For this review, take the finished solid that the model builds, in its own axes (mm). A direction names the side the tool comes from. Round coordinates to 2 decimals unless told otherwise and drop trailing zeros. Write each loop counter-clockwise with the first axis right and the second up, starting at its lowest first coordinate (ties: lowest second). Pieces come first, ordered by that corner, then holes. Notation, with made-up numbers: (-11.75, 48) -> (-1.75, 48) arc R29 ccw to (-1.75, 80) -> close; hole circle Ø5 at (64, 63.25). An arc over 180 degrees is marked (long way). Answer as CSV lines item,"result". Start each with the question number.
Item 1: Machinability: for faces 1 (the flat face through (-12, -1, 4.5)), 2 (the conical face through (-38.13, -18.06, 7.87)), 3 (the cylindrical face through (-28.784, 16.818, 2.885)), which of the approach directions +Z, -Z, +X, -X, +Y, -Y give a long, thin tool a straight path to every point of the face, cutting with its end or side? Answer none if there is none.
Item 2: For pin 1 Ø3 at (y, z) = (12, 4) entering from -X; pin 2 Ø2.5 at (x, z) = (30, 4) entering from +Y; pin 3 Ø4 at (x, y) = (-15, -2) entering from -Z, all flat-tipped, find the tip position at first contact; note any pin that passes through.
Item 3: Mouldability with a two-part tool opening along X and no side actions: class faces 4 (the cylindrical face through (0.4, 13.9, 5.6)), 5 (the conical face through (38.06, -18.13, 7.87)), 6 (the conical face through (-38.12, -18.06, 0.12)), 7 (the cylindrical face through (-18, 0, 6)) as +X half, -X half, draft (parallel to the pull), parting line (faces both ways), or undercut.
Item 4: Take a section at B-B on x = 15. Give the boundary of the cut face in (y, z), then the cut area to 3 significant figures.
Item 5: Wall thickness on probe 1 along X at (y, z) = (13.75, 4); probe 2 along Y at (x, z) = (-15, 1.8); probe 3 along X at (y, z) = (-0.5, 6.25): over which ranges is each line inside the solid? List them lowest first. Write a range as from..to.
Item 6: Take a section at A-A on y = 0. Count the separate pieces of the cut face and the enclosed holes in it, then the cut area to 3 significant figures.
```python
from build123d import *

# Parameters (mm, degrees)
SKETCH1_W                             = 80
SKETCH1_H                             = 40
SKETCH1_R                             = 7
SKETCH1_R_2                           = 3
BOSS_EXTRUDE1_DEPTH                   = 8
CUT_EXTRUDE1_OUTLINE_R                = 7
CUT_EXTRUDE1_OUTLINE_R_2              = 3
CUT_EXTRUDE1_DEPTH                    = 4.5
FILLET1_R                             = 5
TAP_DRILL_FOR_M4X0_7_TAP1_D           = 3.3
TAP_DRILL_FOR_M4X0_7_TAP1_DEPTH       = 12
TAP_DRILL_FOR_M4X0_7_TAP1_CSINK_D     = 3.35
TAP_DRILL_FOR_M4X0_7_TAP1_CSINK_ANGLE = 90
TAP_DRILL_FOR_M4X0_7_TAP1_TIP         = 0.991420021
TAP_DRILL_FOR_M4X0_7_TAP2_D           = 3.3
TAP_DRILL_FOR_M4X0_7_TAP2_DEPTH       = 12
TAP_DRILL_FOR_M4X0_7_TAP2_CSINK_D     = 3.35
TAP_DRILL_FOR_M4X0_7_TAP2_CSINK_ANGLE = 90
TAP_DRILL_FOR_M4X0_7_TAP2_TIP         = 0.991420021
TAP_DRILL_FOR_M4X0_7_TAP3_D           = 3.3
TAP_DRILL_FOR_M4X0_7_TAP3_DEPTH       = 12
TAP_DRILL_FOR_M4X0_7_TAP3_CSINK_D     = 3.35
TAP_DRILL_FOR_M4X0_7_TAP3_CSINK_ANGLE = 90
TAP_DRILL_FOR_M4X0_7_TAP3_TIP         = 0.991420021
CHAMFER1_SIZE                         = 0.75


# Read off the part's stored shape, not the designer's step: Cut-Extrude1
with BuildPart() as part:
    # Sketch1 → Boss-Extrude1 (new body)
    # profile 1 of 3: a face of its own
    with BuildSketch(Plane.XY):
        Rectangle(SKETCH1_W, SKETCH1_H)
        with Locations((15, 0)):
            Circle(SKETCH1_R, mode=Mode.SUBTRACT)
        with Locations((-15, 0)):
            Circle(SKETCH1_R, mode=Mode.SUBTRACT)
    # profile 2 of 3: a face of its own
    with BuildSketch(Plane.XY):
        with Locations((-15, 0)):
            Circle(SKETCH1_R)
        with Locations((-15, 0)):
            Circle(SKETCH1_R_2, mode=Mode.SUBTRACT)
    # profile 3 of 3: a face of its own
    with BuildSketch(Plane.XY):
        with Locations((15, 0)):
            Circle(SKETCH1_R)
        with Locations((15, 0)):
            Circle(SKETCH1_R_2, mode=Mode.SUBTRACT)
    extrude(amount=BOSS_EXTRUDE1_DEPTH)

    # Cut-Extrude1 outline → Cut-Extrude1 (cut)
    # profile 1 of 2: a face of its own
    with BuildSketch(Plane.XY):
        with Locations((-15, 0)):
            Circle(CUT_EXTRUDE1_OUTLINE_R)
        with Locations((-15, 0)):
            Circle(CUT_EXTRUDE1_OUTLINE_R_2, mode=Mode.SUBTRACT)
    # profile 2 of 2: a face of its own
    with BuildSketch(Plane.XY):
        with Locations((15, 0)):
            Circle(CUT_EXTRUDE1_OUTLINE_R)
        with Locations((15, 0)):
            Circle(CUT_EXTRUDE1_OUTLINE_R_2, mode=Mode.SUBTRACT)
    extrude(amount=CUT_EXTRUDE1_DEPTH, mode=Mode.SUBTRACT)

    # Fillet1
    fillet1_edges = [part.edges().sort_by_distance(p)[0] for p in [
        (40, -20, 4),
        (-40, -20, 4),
        (-40, 20, 4),
        (40, 20, 4),
    ]]
    fillet(fillet1_edges, radius=FILLET1_R)

    # Tap Drill for M4x0.7 Tap1
    with Locations(Plane(origin=(0, 20, 0), x_dir=(1, 0, 0), z_dir=(0, 1, 0))):
        with Locations((30, -4), (0, -4), (-30, -4)):
            CounterSinkHole(TAP_DRILL_FOR_M4X0_7_TAP1_D / 2, TAP_DRILL_FOR_M4X0_7_TAP1_CSINK_D / 2, depth=TAP_DRILL_FOR_M4X0_7_TAP1_DEPTH, counter_sink_angle=TAP_DRILL_FOR_M4X0_7_TAP1_CSINK_ANGLE)
            with Locations((0, 0, -(TAP_DRILL_FOR_M4X0_7_TAP1_DEPTH + TAP_DRILL_FOR_M4X0_7_TAP1_TIP / 2))):  # 118° drill point
                Cone(0, TAP_DRILL_FOR_M4X0_7_TAP1_D / 2, TAP_DRILL_FOR_M4X0_7_TAP1_TIP, mode=Mode.SUBTRACT)

    # Tap Drill for M4x0.7 Tap2
    with Locations(Plane(origin=(40, 0, 0), x_dir=(0, 0, -1), z_dir=(1, 0, 0))):
        with Locations((-4, 12)):
            CounterSinkHole(TAP_DRILL_FOR_M4X0_7_TAP2_D / 2, TAP_DRILL_FOR_M4X0_7_TAP2_CSINK_D / 2, depth=TAP_DRILL_FOR_M4X0_7_TAP2_DEPTH, counter_sink_angle=TAP_DRILL_FOR_M4X0_7_TAP2_CSINK_ANGLE)
            with Locations((0, 0, -(TAP_DRILL_FOR_M4X0_7_TAP2_DEPTH + TAP_DRILL_FOR_M4X0_7_TAP2_TIP / 2))):  # 118° drill point
                Cone(0, TAP_DRILL_FOR_M4X0_7_TAP2_D / 2, TAP_DRILL_FOR_M4X0_7_TAP2_TIP, mode=Mode.SUBTRACT)

    # Tap Drill for M4x0.7 Tap3
    with Locations(Plane.ZY.offset(40)):
        with Locations((4, 12)):
            CounterSinkHole(TAP_DRILL_FOR_M4X0_7_TAP3_D / 2, TAP_DRILL_FOR_M4X0_7_TAP3_CSINK_D / 2, depth=TAP_DRILL_FOR_M4X0_7_TAP3_DEPTH, counter_sink_angle=TAP_DRILL_FOR_M4X0_7_TAP3_CSINK_ANGLE)
            with Locations((0, 0, -(TAP_DRILL_FOR_M4X0_7_TAP3_DEPTH + TAP_DRILL_FOR_M4X0_7_TAP3_TIP / 2))):  # 118° drill point
                Cone(0, TAP_DRILL_FOR_M4X0_7_TAP3_D / 2, TAP_DRILL_FOR_M4X0_7_TAP3_TIP, mode=Mode.SUBTRACT)

    # Chamfer1
    chamfer1_edges = [part.edges().sort_by_distance(p)[0] for p in [
        (8, 0, 0),
        (-18, 0, 8),
        (-22, 0, 0),
        (12, 0, 8),
        (40, 0, 0),
        (40, 0, 8),
        (0, -20, 0),
        (-40, 0, 0),
        (0, 20, 0),
        (38.535533906, 18.535533906, 0),
        (-38.535533906, 18.535533906, 0),
        (-38.535533906, -18.535533906, 0),
        (38.535533906, -18.535533906, 0),
        (0, -20, 8),
        (0, 20, 8),
        (-40, 0, 8),
        (38.535533906, 18.535533906, 8),
        (-38.535533906, 18.535533906, 8),
        (-38.535533906, -18.535533906, 8),
        (38.535533906, -18.535533906, 8),
    ]]
    chamfer(chamfer1_edges, length=CHAMFER1_SIZE)


solid = part.part
```
Output values:
1,face 1,"-Z"
1,face 2,"+Z, -X, -Y"
1,face 3,"+Y"
2,pin 1,"stops at x = -27.91"
2,pin 2,"stops at y = 7.76"
2,pin 3,"stops at z = 4.5"
3,face 4,"undercut"
3,face 5,"+X half"
3,face 6,"-X half"
3,face 7,"undercut"
4,outline,"(-20, 0.75) -> (-19.25, 0) -> (-7.75, 0) -> (-7, 0.75) -> (-7, 4.5) -> (-3, 4.5) -> (-3, 7.25) -> (-3.75, 8) -> (-19.25, 8) -> (-20, 7.25) -> close; (3, 4.5) -> (7, 4.5) -> (7, 0.75) -> (7.75, 0) -> (19.25, 0) -> (20, 0.75) -> (20, 7.25) -> (19.25, 8) -> (3.75, 8) -> (3, 7.25) -> close"
4,area,"234 mm^2"
5,probe 1,"x = -40..-31.65, -28.35..-1.65, 1.65..28.35, 31.65..40"
5,probe 2,"y = -20..-7, 7..20"
5,probe 3,"x = -40..-17.96, -12.04..12.04, 17.96..40"
6,separate pieces,"3"
6,enclosed holes,"0"
6,area,"469 mm^2"
